Input: part model. Units: mm. Frame: model coordinates. Coordinates: 2 decimals unless noted, no trailing zeros. Order: outer loops, then holes, each group sorted by start corner. A loop starts at its lowest first (then second) coordinate and runs counter-clockwise, first axis right, second up. Notation, with made-up numbers: (77.25, 9.5) -> (124.25, 9.5) arc R13 cw to (124.25, 31.5) -> close; hole circle Ø10 at (25.25, -28). An arc over 180 degrees is marked (long way). Answer as CSV lines item,"result".
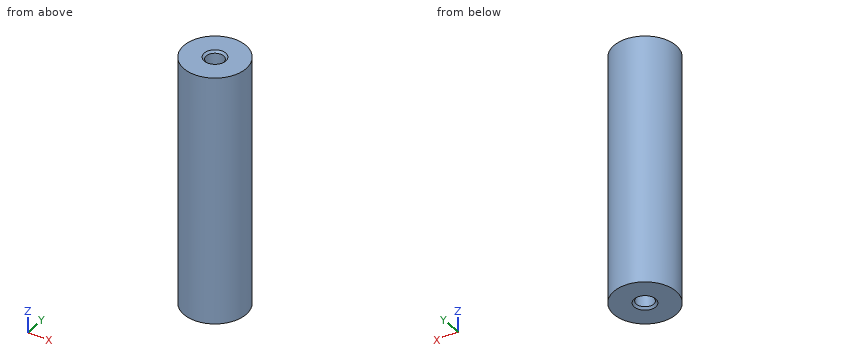
Solid Edge part; units mm, degrees
sketch "Sketch1" plane through (0, 0, 0) normal (0, 0, 1) x (1, 0, 0)
  circle A0 centre (0, 0) radius 15
extrude "Protrusion1" add sketch "Sketch1" along normal blind 120
hole "Gewinde_oben" at (0, 0, 120) direction (0, 0, -1) diameter 8.376 depth 35 start chamfer 1 start chamfer angle 45
hole "Gewinde_unten" at (0, 0, 0) direction (0, 0, 1) diameter 8.376 depth 35 start chamfer 1 start chamfer angle 45
1. Ray query, line 1 along Y through (x, z) = (0, 103); line 2 along X through (y, z) = (-0.5, 71.5); line 3 along X through (y, z) = (2, 115). Return the intervals inside material, ascending.
Findings:
line 1,"y = -15 to -4.19, 4.19 to 15"
line 2,"x = -14.99 to 14.99"
line 3,"x = -14.87 to -3.68, 3.68 to 14.87"
2. Cut plane D-D (z = 49). Return the cut outline in (x, y), plus the area to 3 significant figures.
Findings:
outline,"circle Ø30 at (0, 0)"
area,"707 mm2"
3. Cut plane A-A (y = 0). Return the cut outline in (x, z), plus the area to 3 significant figures.
Findings:
outline,"(-15, 0) -> (-5.19, 0) -> (-4.19, 1) -> (-4.19, 35) -> (4.19, 35) -> (4.19, 1) -> (5.19, 0) -> (15, 0) -> (15, 120) -> (5.19, 120) -> (4.19, 119) -> (4.19, 85) -> (-4.19, 85) -> (-4.19, 119) -> (-5.19, 120) -> (-15, 120) -> close"
area,"3,010 mm2"
4. Cut plane C-C (z = 96.5). Return the cut outline in (x, y).
Findings:
outline,"circle Ø30 at (0, 0); hole circle Ø8.38 at (0, 0)"
5. Contact query for flat-ended pins moving along their axis: pin 1 (2.5 mm diameter, centred on x = -0.5, y = 0.5, fed in from -Z); pin 2 (4 mm diameter, centred on x = 8, z = 15.5, fed in from +Y); pin 3 (2 mm diameter, centred on y = -3.5, z = 67, fed in from +X). Output: stop coordinate, or through.
Findings:
pin 1,"stops at z = 35"
pin 2,"stops at y = 13.75"
pin 3,"stops at x = 14.79"
